Source: CAD feature listing. Evaluate the final solid. Frame: model axes, mm. A direction names the side the tool comes from. Coordinates: 2 decimals unless noted, no trailing zeros. Order: outer loops, then holes, each group sorted by start corner. A loop starts at its lowest first (then second) coordinate and runs counter-clockwise, first axis right, second up.
Item 1: Contact query for flat-ended pins moving along their axis: P1, Ø8, axis at y = 0, z = 10.5, coming from the -X side; P2, Ø2, axis at y = 10, z = 20, coming from the +X side; P3, Ø8, axis at x = 18.5, z = 14.5, coming from the -Y side; P4, Ø8, axis at x = 3, y = -15, coming from the -Z side. Output: stop coordinate, or through.
Item 2: Mould query, pull axis Y, two halves, no side actions, for faces 1 (the flat face through (11, 11, 1.2)), 2 (the flat face through (0, 0, 25)), 3 (the cylindrical face through (-20.395, 15.638, 0.592)). Classes: released by +Y, released by -Y, zero draft, split by the parting line, or undercut.
Item 3: Section D-D on x = -18. Return the cut outline in (y, z).
Item 4: Section C-C on z = 13.25. Return the cut outline in (x, y).
Item 5: Section A-A on x = 0. Return the cut outline in (y, z), then the cut area to 3 significant figures.
Item 6: Ray query, line 1 (Y direction, x = 0, z = 13.5); line 2 (Z direction, x = -14.5, y = 13); line 3 (Y direction, x = 3, z = 6.75). Return the intervals inside material, ascending.
Item 7: Reachability of faces 4 (the cylindrical face through (11.923, 3.755, 12.325)), 5 (the cylindrical face through (-10.097, 9.259, 13.673)), 6 (the flat face through (0, 0, 26.5)) from +Z, -Z, +X, -X, +Y, -Y: full face, straight path, thin tool, end or side. Return the list, or none.
from build123d import *

# Parameters (mm, degrees)
F0_R     = 13.7
F0_R_2   = 12.5
F1_DEPTH = 25
F2_R     = 13.7
F3_DEPTH = 1.5
F4_R     = 25.7
F4_R_2   = 13.7
F5_DEPTH = 1.2


with BuildPart() as f1:
    # F0 (on Top) → F1 (new body)
    with BuildSketch(Plane.XY):
        Circle(F0_R)
        Circle(F0_R_2, mode=Mode.SUBTRACT)
    extrude(amount=F1_DEPTH)

    # F2 (on face) → F3 (join)
    with BuildSketch(Plane.XY.offset(25)):
        Circle(F2_R)
    extrude(amount=F3_DEPTH)

    # F4 (on face) → F5 (join)
    with BuildSketch(Plane(origin=(0, 0, 0), x_dir=(1, 0, 0), z_dir=(0, 0, -1))):
        Circle(F4_R)
        Circle(F4_R_2, mode=Mode.SUBTRACT)
    extrude(amount=-F5_DEPTH)


solid = f1.part
Answer list:
1. P1: stops at x = -13.7
1. P2: stops at x = 10.33
1. P3: passes through
1. P4: stops at z = 0
2. face 1: zero draft
2. face 2: undercut
2. face 3: split by the parting line
3. outline: (-18.34, 0) - (18.34, 0) - (18.34, 1.2) - (-18.34, 1.2) - close
4. outline: circle Ø27.4 at (0, 0); hole circle Ø25 at (0, 0)
5. outline: (-25.7, 0) - (-12.5, 0) - (-12.5, 25) - (12.5, 25) - (12.5, 0) - (25.7, 0) - (25.7, 1.2) - (13.7, 1.2) - (13.7, 26.5) - (-13.7, 26.5) - (-13.7, 1.2) - (-25.7, 1.2) - close
5. area: 130 mm2
6. line 1: y = -13.7 to -12.5, 12.5 to 13.7
6. line 2: z = 0 to 1.2
6. line 3: y = -13.37 to -12.13, 12.13 to 13.37
7. face 4: -Z
7. face 5: +Z
7. face 6: +Z, +X, -X, +Y, -Y
